Geometry: final body of the model. Coordinates: model frame, mm. A direction names the side the tool comes from. Give positions to 0.01 mm unless a question says otherwise; leave off trailing zeros. Order: outer loops, then holes, each group sorted by start corner. A loop starts at its lowest first (then second) coordinate and runs counter-clockwise, first axis right, second up. Notation, with made-up numbers: M 78,-1.5 L 135,-1.5 A23 cw 135,17.5 Z; hole C -36,24.5 d10. An arc over 180 degrees is marked long. Use CSV: the item, a comma, the result in double quotes.
```python
from build123d import *

# Parameters (mm, degrees)
SKETCH3_R           = 48.895
BOSS_EXTRUDE2_DEPTH = 5.08
SKETCH4_R           = 42.9006
BOSS_EXTRUDE3_DEPTH = 15.24
SKETCH5_R           = 48.895
SKETCH5_R_2         = 46.609
BOSS_EXTRUDE4_DEPTH = 38.1
CUT_EXTRUDE1_DEPTH  = 0.2


with BuildPart() as part:
    # Sketch3 → Boss-Extrude2 (new body)
    with BuildSketch(Plane(origin=(0, 0, 0), x_dir=(1, 0, 0), z_dir=(0, 1, 0))):
        with Locations(Location((0, 0, 0), (0, 0, 270))):  # turned: the seam where the file's is
            Circle(SKETCH3_R)
    extrude(amount=BOSS_EXTRUDE2_DEPTH)

    # Sketch4 → Boss-Extrude3 (add)
    with BuildSketch(Plane(origin=(0, 5.08, 0), x_dir=(1, 0, 0), z_dir=(0, 1, 0))):
        with Locations(Location((0, 0, 0), (0, 0, 270))):  # turned: the seam where the file's is
            Circle(SKETCH4_R)
        with BuildLine():
            ThreePointArc((-4.567935909, -12.199290546), (-0.649198876, -13.01027552), (3.330805622, -12.593429326))
            Line((3.330805622, -12.593429326), (9.293981813, -22.921953464))
            Line((9.293981813, -22.921953464), (14.133331769, -20.127953464))
            Line((14.133331769, -20.127953464), (8.306068354, -10.034837158))
            ThreePointArc((8.306068354, -10.034837158), (11.129081005, -6.769954526), (12.730314912, -2.761849113))
            Line((12.730314912, -2.761849113), (24.159656791, -2.761849113))
            Line((24.159656791, -2.761849113), (24.159656791, 2.826150887))
            Line((24.159656791, 2.826150887), (12.716194378, 2.826150887))
            ThreePointArc((12.716194378, 2.826150887), (11.103422614, 6.811955266), (8.280927567, 10.055593813))
            Line((8.280927567, 10.055593813), (14.133331769, 20.192255238))
            Line((14.133331769, 20.192255238), (9.293981813, 22.986255238))
            Line((9.293981813, 22.986255238), (3.298576906, 12.601909327))
            ThreePointArc((3.298576906, 12.601909327), (-0.649560207, 13.010257485), (-4.537389725, 12.210684779))
            Line((-4.537389725, 12.210684779), (-10.758668231, 22.986255238))
            Line((-10.758668231, 22.986255238), (-15.598018187, 20.192255238))
            Line((-15.598018187, 20.192255238), (-9.240826906, 9.181276947))
            ThreePointArc((-9.240826906, 9.181276947), (-11.429112071, 6.250130044), (-12.716194378, 2.826150887))
            Line((-12.716194378, 2.826150887), (-25.624343209, 2.826150887))
            Line((-25.624343209, 2.826150887), (-25.624343209, -2.761849113))
            Line((-25.624343209, -2.761849113), (-12.730314912, -2.761849113))
            ThreePointArc((-12.730314912, -2.761849113), (-11.452817768, -6.206584686), (-9.26428516, -9.15760606))
            Line((-9.26428516, -9.15760606), (-15.598018187, -20.127953464))
            Line((-15.598018187, -20.127953464), (-10.758668231, -22.921953464))
            Line((-10.758668231, -22.921953464), (-4.567935909, -12.199290546))
        make_face(mode=Mode.SUBTRACT)
    extrude(amount=BOSS_EXTRUDE3_DEPTH)

    # Sketch5 → Boss-Extrude4 (add)
    with BuildSketch(Plane(origin=(0, 5.08, 0), x_dir=(1, 0, 0), z_dir=(0, 1, 0))):
        with Locations(Location((0, 0, 0), (0, 0, 270))):  # turned: the seam where the file's is
            Circle(SKETCH5_R)
        with Locations(Location((0, 0, 0), (0, 0, 270))):  # turned: the seam where the file's is
            Circle(SKETCH5_R_2, mode=Mode.SUBTRACT)
    extrude(amount=BOSS_EXTRUDE4_DEPTH)

    # Sketch7 → Cut-Extrude1 (cut)
    with BuildSketch(Plane.XZ):
        with BuildLine():
            Line((10.189077573, 28.777139206), (3.905470201, 28.777139206))
            add(Edge.make_bspline(
                [(3.905470201, 28.777139206), (5.673403675, 10.082176027), (2.072299934, -8.408708001)],
                knots=[0, 0, 0, 1, 1, 1], degree=2))
            Line((2.072299934, -8.408708001), (1.578207561, -8.290715793))
            Line((1.578207561, -8.290715793), (0.93540787, -10.43338143))
            add(Edge.make_bspline(
                [(0.93540787, -10.43338143), (-1.730658467, -9.24791296), (-2.648379288, -6.465006437)],
                knots=[0, 0, 0, 1, 1, 1], degree=2))
            add(Edge.make_bspline(
                [(-1.535058391, -14.046142711), (-3.997790421, -10.512351861), (-2.648379288, -6.465006437)],
                knots=[0, 0, 0, 1, 1, 1], degree=2))
            add(Edge.make_bspline(
                [(-5.496336768, -32.152202336), (-5.134044818, -22.716243693), (-1.535058391, -14.046142711)],
                knots=[0, 0, 0, 1, 1, 1], degree=2))
            add(Edge.make_bspline(
                [(-3.921713234, -32.261214734), (-5.591404908, -34.721729292), (-5.496336768, -32.152202336)],
                knots=[0, 0, 0, 1, 1, 1], degree=2))
            add(Edge.make_bspline(
                [(-3.921713234, -32.261214734), (0.67700242, -24.157422119), (3.257772607, -15.187585129)],
                knots=[0, 0, 0, 1, 1, 1], degree=2))
            add(Edge.make_bspline(
                [(3.257772607, -15.187585129), (7.244573316, -13.614377412), (9.294943691, -9.762880676)],
                knots=[0, 0, 0, 1, 1, 1], degree=2))
            add(Edge.make_bspline(
                [(3.445088013, -11.186285473), (6.51327774, -11.392596023), (9.294943691, -9.762880676)],
                knots=[0, 0, 0, 1, 1, 1], degree=2))
            Line((3.445088013, -11.186285473), (4.130880832, -8.90030941))
            Line((4.130880832, -8.90030941), (3.845040397, -8.832049008))
            add(Edge.make_bspline(
                [(10.189077573, 28.777139206), (10.494453194, 9.291070289), (3.845040397, -8.832049008)],
                knots=[0, 0, 0, 1, 1, 1], degree=2))
        make_face()
    extrude(amount=-CUT_EXTRUDE1_DEPTH, mode=Mode.SUBTRACT)


solid = part.part
```
1. Section B-B, the plane x = -39. Return the cut outline in (y, z).
Answer:
outline,"M 0,-29.49 L 43.18,-29.49 L 43.18,-25.52 L 5.08,-25.52 L 5.08,-17.87 L 20.32,-17.87 L 20.32,17.87 L 5.08,17.87 L 5.08,25.52 L 43.18,25.52 L 43.18,29.49 L 0,29.49 Z"
2. Line query: line 1 (X direction, y = 31, z = 0) (3 decimals); line 2 (X direction, y = 12, z = -32.5); line 3 (Z direction, x = -8, y = 12.5). Output: solid intervals per line, ascending.
Answer:
line 1,"-48.895 to -46.609, 46.609 to 48.895"
line 2,"-36.53 to -33.41, -28 to 28, 33.41 to 36.53"
line 3,"-48.24 to -45.92, -42.15 to -18.21, 18.14 to 42.15, 45.92 to 48.24"
3. Section A-A, the plane y = 6.5. Return the cut outline in (x, z) (3 decimals), plus the area to 3 significant figures.
Answer:
outline,"C 0,0 d97.79; C 0,0 d85.801; hole C 0,0 d93.218; hole M -25.624,-2.826 L -12.716,-2.826 A13.026 ccw -9.241,-9.181 L -15.598,-20.192 L -10.759,-22.986 L -4.537,-12.211 A13.026 ccw 3.299,-12.602 L 9.294,-22.986 L 14.133,-20.192 L 8.281,-10.056 A13.026 ccw 12.716,-2.826 L 24.16,-2.826 L 24.16,2.762 L 12.73,2.762 A13.026 ccw 8.306,10.035 L 14.133,20.128 L 9.294,22.922 L 3.331,12.593 A13.026 ccw -4.568,12.199 L -10.759,22.922 L -15.598,20.128 L -9.264,9.158 A13.026 ccw -12.73,2.762 L -25.624,2.762 Z"
area,"5,530 mm2"
4. Pin query (flat end, axial travel): pin 1 Ø6.5 at (x, y) = (-22, 15.5) entering from +Z; pin 2 Ø23 at (x, z) = (5.5, -6) entering from +Y; pin 3 Ø12 at (x, y) = (32.5, 25) entering from -Z. Return the tip coordinate at first contact, or that it passes through.
Answer:
pin 1,"z = 45.16"
pin 2,"y = 20.32"
pin 3,"z = -41.09"
5. Reachability of faces 4 (the face through (-12.46, 12.59, -14.76)), 5 (the face through (4, 0.2, 0)) from +Z, -Z, +X, -X, +Y, -Y: full face, straight path, thin tool, end or side. Return the list, or none.
Answer:
face 4,"+Y"
face 5,"-Y"
6. Section D-D, the plane z = 41. Return the cut outline in (x, y), plus the area to 3 significant figures.
Answer:
outline,"M -26.64,0 L 26.64,0 L 26.64,43.18 L 22.17,43.18 L 22.17,5.08 L 12.63,5.08 L 12.63,20.32 L -12.63,20.32 L -12.63,5.08 L -22.17,5.08 L -22.17,43.18 L -26.64,43.18 Z"
area,"996 mm2"
7. Pull-direction query (Z, two-part tool) for faces 1 (the face through (1, 0, -1)), 2 (the face through (-47.732, 21.288, -10.599)), 3 (the face through (-11.4, 12.6, -6.3)); classes: +Z half, -Z half, draft (parallel to the pull), parting line (faces both ways), or undercut.
Answer:
face 1,"draft"
face 2,"parting line"
face 3,"undercut"
8. Section C-C, the plane y = 37. Return the cut outline in (x, z) (3 decimals), plus the area to 3 significant figures.
Answer:
outline,"C 0,0 d97.79; hole C 0,0 d93.218"
area,"686 mm2"
